from build123d import *

# Parameters (mm, degrees)
SKETCH1_W           = 59
SKETCH1_H           = 36
BOSS_EXTRUDE1_DEPTH = 17.5
SKETCH2_W           = 53
SKETCH2_H           = 30
CUT_EXTRUDE1_DEPTH  = 15.9
SKETCH3_OUTSIDE_W   = 75.26
SKETCH3_OUTSIDE_H   = 52.26
SKETCH3_OUTSIDE_W_2 = 55.8
SKETCH3_OUTSIDE_H_2 = 32.8
CUT_EXTRUDE2_DEPTH  = 15.5
CUT_EXTRUDE3_DEPTH  = 1.4
FILLET1_R           = 1


with BuildPart() as part:
    # Sketch1 → Boss-Extrude1 (new body)
    with BuildSketch(Plane(origin=(0, 0, 0), x_dir=(1, 0, 0), z_dir=(0, 1, 0))):
        Rectangle(SKETCH1_W, SKETCH1_H)
    extrude(amount=BOSS_EXTRUDE1_DEPTH)

    # Sketch2 → Cut-Extrude1 (cut)
    with BuildSketch(Plane.XZ):
        Rectangle(SKETCH2_W, SKETCH2_H)
    extrude(amount=-CUT_EXTRUDE1_DEPTH, mode=Mode.SUBTRACT)

    # Sketch3 outside → Cut-Extrude2 (cut)
    with BuildSketch(Plane(origin=(0, 17.5, 0), x_dir=(1, 0, 0), z_dir=(0, 1, 0))):
        Rectangle(SKETCH3_OUTSIDE_W, SKETCH3_OUTSIDE_H)
        Rectangle(SKETCH3_OUTSIDE_W_2, SKETCH3_OUTSIDE_H_2, mode=Mode.SUBTRACT)
    extrude(amount=-CUT_EXTRUDE2_DEPTH, mode=Mode.SUBTRACT)

    # Sketch4 → Cut-Extrude3 (cut)
    with BuildSketch(Plane(origin=(27.9, 0, 0), x_dir=(0, 0, -1), z_dir=(1, 0, 0))):
        with BuildLine():
            Line((2.25, 16), (-2.5, 16))
            ThreePointArc((-2.5, 16), (-4.9, 13.6), (-2.5, 11.2))
            Line((-2.5, 11.2), (2.25, 11.2))
            ThreePointArc((2.25, 11.2), (4.65, 13.6), (2.25, 16))
        make_face()
    extrude(amount=-CUT_EXTRUDE3_DEPTH, mode=Mode.SUBTRACT)

    # Fillet1
    fillet1_edges = [part.edges().sort_by_distance(p)[0] for p in [
        (-29.5, 1, -18),
        (29.5, 1, -18),
        (0, 2, -18),
        (29.5, 1, 18),
        (-29.5, 1, 18),
        (-29.5, 2, 0),
        (0, 2, 18),
        (29.5, 2, 0),
        (-27.9, 17.5, 0),
        (-27.9, 9.75, -16.4),
        (0, 17.5, -16.4),
        (27.9, 9.75, -16.4),
        (27.9, 17.5, 0),
        (27.9, 9.75, 16.4),
        (0, 17.5, 16.4),
        (-27.9, 9.75, 16.4),
        (0, 0, -18),
        (29.5, 0, 0),
        (0, 0, 18),
        (-29.5, 0, 0),
    ]]
    fillet(fillet1_edges, radius=FILLET1_R - 0.0001)  # a hair under: the kernel refuses the full size


solid = part.part
Input: part model. Units: mm. Frame: model coordinates. A direction names the side the tool comes from. Coordinates: 2 decimals unless noted, no trailing zeros. Write each loop counter-clockwise with the first axis right and the second up, starting at its lowest first coordinate (ties: lowest second). Pieces come first, ordered by that corner, then holes. Notation, with made-up numbers: M 1,18 L 11,18 A32 cw 11,47 Z; hole C -20.75,65 d5. An arc over 180 degrees is marked long. Answer as a JSON object with one key per item and string values. Group by question number.
(1) Set-up query: faces 4 (the face through (27, 11.2, 0)), 5 (the face through (27.9, 9, 0)), 6 (the face through (0, 9, -16.4)), 7 (the face through (0, 9, 16.4)), 8 (the face through (-26.5, 8, 0)). Return all of +Z, -Z, +X, -X, +Y, -Y with unobstructed straight access to the full face (end or side cutting, diameter ignored); none if empty.
(2) Contact query for flat-ended pins moving along their axis: P1, Ø5, axis at y = 9, z = 13.5, coming from the -X side; P2, Ø10, axis at x = -23, y = 10, coming from the +Z side; P3, Ø5, axis at y = 4, z = -5.5, coming from the -X side. Output: stop coordinate, or through.
(3) Mould query, pull axis Y, two halves, no side actions, for faces 1 (the face through (0, 8, -15)), 2 (the face through (0, 17.5, 0)), 3 (the face through (27, 16, 0)). Classes: pulls with the +Y half, pulls with the -Y half, needs draft (parallel to the pull), parting line crosses it, or undercut.
(4) Section A-A on y = 6.5. Output: boundary loops of the cut face in (x, z), plus the area to 3 significant figures.
(5) Ray query, line 1 along Z through (x, y) = (-21.5, 12.75); line 2 along X through (y, z) = (11, -8); line 3 along Y through (x, z) = (19.5, 3.5). Return the intervals inside material, ascending. Write a range as [from, to].
(6) Section D-D on y = 13.6. Output: boundary loops of the cut face in (x, z).
Result set:
{
 "1": {"face 4": "+X", "face 5": "+Z, -Z, +X, +Y", "face 6": "-Z, +X, -X, +Y", "face 7": "+Z, +X, -X, +Y", "face 8": "-Y"},
 "2": {"P1": "stops at x = -27.9", "P2": "stops at z = 16.4", "P3": "stops at x = -29.37"},
 "3": {"face 1": "needs draft", "face 2": "pulls with the +Y half", "face 3": "undercut"},
 "4": {"outline": "M -27.9,-15.4 A1 ccw -26.9,-16.4 L 26.9,-16.4 A1 ccw 27.9,-15.4 L 27.9,15.4 A1 ccw 26.9,16.4 L -26.9,16.4 A1 ccw -27.9,15.4 Z; hole M -26.5,-15 L 26.5,-15 L 26.5,15 L -26.5,15 Z", "area": "239 mm2"},
 "5": {"line 1": "z = [-16.4, -15], [15, 16.4]", "line 2": "x = [-27.9, -26.5], [26.5, 27.9]", "line 3": "y = [15.9, 17.5]"},
 "6": {"outline": "M -27.9,-15.4 A1 ccw -26.9,-16.4 L 26.9,-16.4 A1 ccw 27.9,-15.4 L 27.9,-4.65 L 26.5,-4.65 L 26.5,-15 L -26.5,-15 L -26.5,15 L 26.5,15 L 26.5,4.9 L 27.9,4.9 L 27.9,15.4 A1 ccw 26.9,16.4 L -26.9,16.4 A1 ccw -27.9,15.4 Z"}
}
